Autodesk Inventor part; units mm, degrees
ref_plane "YZ Plane" through (0, 0, 0) normal (1, 0, 0) x (0, 1, 0)
ref_plane "XZ Plane" through (0, 0, 0) normal (0, 1, 0) x (-1, 0, 0)
ref_plane "XY Plane" through (0, 0, 0) normal (0, 0, 1) x (1, 0, 0)
sketch "Sketch1" plane through (0, 0, 0) normal (0, 1, 0) x (-1, 0, 0)
  line L0 (-0.4496, -29.3) -> (-0.4496, 0)
  line L1 (-41.2289, 0) -> (-41.2289, -29.3)
  circle A0 centre (-49.9386, -23.2) radius 1.05
  circle A1 centre (-50.9386, -9.98) radius 1.05
  circle A2 centre (-57.9386, -2.68) radius 1.05
  circle A3 centre (-64.9386, -9.98) radius 1.05
  circle A4 centre (-65.9386, -23.2) radius 1.05
  circle A5 centre (23.785, -2.5) radius 1.05
  circle A6 centre (8.735, -2.5) radius 1.05
  circle A7 centre (23.785, -17.6) radius 1.05
  circle A8 centre (8.735, -17.6) radius 1.05
  circle A9 centre (-25.6393, -7) radius 1.55
  circle A10 centre (-35.7793, -7) radius 1.55
  circle A11 centre (-25.6393, -22.3) radius 1.55
  circle A12 centre (-35.7793, -22.3) radius 1.55
  arc A13 (-67.0086, 0) -> (-68.0086, -1) centre (-67.0086, -1) ccw
  line L2 (-67.0086, 0) -> (25.33, 0)
  line L3 (-68.0086, -28.3) -> (-68.0086, -1)
  arc A14 (-68.0086, -28.3) -> (-67.0086, -29.3) centre (-67.0086, -28.3) ccw
  line L4 (-63.885, -29.3) -> (-67.0086, -29.3)
  arc A15 (-51.9921, -29.3) -> (-63.885, -29.3) centre (-57.9386, -30.1) ccw
  line L5 (10.3136, -29.3) -> (-51.9921, -29.3)
  arc A16 (22.2064, -29.3) -> (10.3136, -29.3) centre (16.26, -30.1) ccw
  line L6 (25.33, -29.3) -> (22.2064, -29.3)
  arc A17 (25.33, -29.3) -> (26.33, -28.3) centre (25.33, -28.3) ccw
  line L7 (26.33, -1) -> (26.33, -28.3)
  arc A18 (26.33, -1) -> (25.33, 0) centre (25.33, -1) ccw
  line L8 (-41.6786, -29.3) -> (-41.6786, 0)
  line L9 (-40.7793, 0) -> (-40.7793, -29.3)
  line L10 (-0.8993, -29.3) -> (-0.8993, 0)
  line L11 (0, 0) -> (0, -29.3)
  point P0 (0, 0)
extrude "Extrusion1" add sketch "Sketch1" against normal blind 1.5
sketch "Sketch2" plane through (0, 0, 0) normal (0, 1, 0) x (1, 0, 0)
  circle A0 centre (-16.26, 30.1) radius 6.75
  circle A1 centre (57.9386, 30.1) radius 6.75
  point P0 (0, 0)
  dimension "d2" = 13.5
  dimension "d3" = 13.5
extrude "Extrusion2" cut sketch "Sketch2" against normal blind 10
properties part number "axis_22_bottom_frame"
The listing builds one solid part. Answer for the finished solid, in the listing's coordinates (mm). Round coordinates to 2 decimals unless told otherwise and drop trailing zeros. Order: outer loops, then holes, each group sorted by start corner. A loop starts at its lowest first (then second) coordinate and runs counter-clockwise, first axis right, second up. Notation, with made-up numbers: (-14, 88.25) -> (24, 88.25) arc R30 ccw to (24, 120.25) -> close; hole circle Ø10 at (80.25, 24). An arc over 180 degrees is marked (long way). Answer as CSV lines item,"result". Start each with the question number.
(1) The part is cut by section A-A (y = -0.9). Count the separate pieces of the cut face and the enclosed holes in it, then the cut area to 3 significant figures.
(2) Find the intervals of material crossed by probe 1 along X at (y, z) = (-0.15, -7.25); probe 2 along X at (y, z) = (-0.75, -24.5); probe 3 along Z at (x, y) = (-9, -1), in increasing order. Write a range as from..to.
(3) A flat-ended cylindrical pin translates along its axis: pin 1 Ø3 at (x, z) = (25.64, -7) entering from +Y. Find the tip coordinate at first contact, or state that the pin passes through.
(4) For a pull along Z with two mould halves and no side action, classify faces 1 (the face through (-22.736, -0.74, -2.454)), 2 (the face through (21, 0, -14)), 3 (the face through (-24, -1, -29.3)), 4 (the face through (65.988, -0.74, -9.934)) as +Z half, -Z half, draft (parallel to the pull), parting line (faces both ways), or undercut.
(5) The part is cut by section B-B (z = -7). Determine the outline of the cut face in (x, y), then the cut area to 3 significant figures.
(6) The part is cut by section C-C (z = -27.5). Determine the outline of the cut face in (x, y).
Evaluation:
1,separate pieces,"1"
1,enclosed holes,"13"
1,area,"2,580 mm²"
2,probe 1,"-26.33..24.11, 27.17..34.25, 37.31..68.01"
2,probe 2,"-26.33..-20.03, -12.49..54.17, 61.71..68.01"
2,probe 3,"-29.3..-18.62, -16.58..-3.52, -1.48..0"
3,pin 1,"through"
4,face 1,"undercut"
4,face 2,"draft"
4,face 3,"-Z half"
4,face 4,"undercut"
5,outline,"(-26.33, -1.5) -> (24.09, -1.5) -> (24.09, 0) -> (-26.33, 0) -> close; (27.19, -1.5) -> (34.23, -1.5) -> (34.23, 0) -> (27.19, 0) -> close; (37.33, -1.5) -> (68.01, -1.5) -> (68.01, 0) -> (37.33, 0) -> close"
5,area,"132 mm²"
6,outline,"(-26.33, -1.5) -> (-22.49, -1.5) -> (-22.49, 0) -> (-26.33, 0) -> close; (-10.03, -1.5) -> (51.71, -1.5) -> (51.71, 0) -> (-10.03, 0) -> close; (64.17, -1.5) -> (68.01, -1.5) -> (68.01, 0) -> (64.17, 0) -> close"
